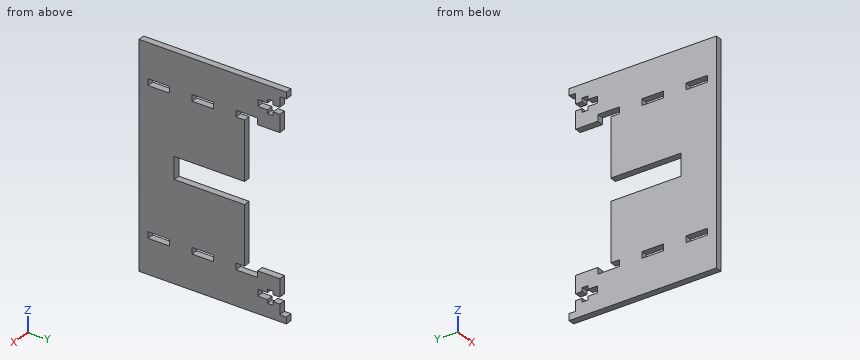
```python
from build123d import *

# Parameters (mm, degrees)
SKETCH1_W           = 100
SKETCH1_H           = 64
BOSS_EXTRUDE1_DEPTH = 3
SKETCH2_W           = 2.9
SKETCH2_H           = 9.8
CUT_EXTRUDE1_DEPTH  = 3
CUT_EXTRUDE2_DEPTH  = 10
SKETCH5_W           = 63
SKETCH5_H           = 16
CUT_EXTRUDE3_DEPTH  = 10
SKETCH6_W           = 10
SKETCH6_H           = 32
CUT_EXTRUDE4_DEPTH  = 10
SKETCH7_W           = 3
SKETCH7_H           = 3
BOSS_EXTRUDE2_DEPTH = 3


with BuildPart() as part:
    # Sketch1 → Boss-Extrude1 (new body)
    with BuildSketch(Plane(origin=(0, 0, 0), x_dir=(0, 0, -1), z_dir=(1, 0, 0))):
        Rectangle(SKETCH1_W, SKETCH1_H)
    extrude(amount=BOSS_EXTRUDE1_DEPTH)

    # Sketch2 → Cut-Extrude1 (cut)
    with BuildSketch(Plane(origin=(3, 0, 0), x_dir=(0, 0, -1), z_dir=(1, 0, 0))):
        with Locations((-32.95, 17)):
            Rectangle(SKETCH2_W, SKETCH2_H)
        with Locations((-32.95, -3)):
            Rectangle(SKETCH2_W, SKETCH2_H)
        with Locations((-32.95, -23)):
            Rectangle(SKETCH2_W, SKETCH2_H)
        with Locations((32.95, -23)):
            Rectangle(SKETCH2_W, SKETCH2_H)
        with Locations((32.95, -3)):
            Rectangle(SKETCH2_W, SKETCH2_H)
        with Locations((32.95, 17)):
            Rectangle(SKETCH2_W, SKETCH2_H)
    extrude(amount=-CUT_EXTRUDE1_DEPTH, mode=Mode.SUBTRACT)

    # Sketch3 → Cut-Extrude2 (cut)
    with BuildSketch(Plane(origin=(3, 0, 0), x_dir=(0, 0, -1), z_dir=(1, 0, 0))):
        Polygon((-42.4, 32), (-42.4, 29), (-44, 29), (-44, 26.4), (-42.4, 26.4), (-42.4, 22), (-39.4, 22), (-39.4, 26.4), (-37.8, 26.4), (-37.8, 29), (-39.4, 29), (-39.4, 32), align=None)
    cut_extrude2 = extrude(amount=-CUT_EXTRUDE2_DEPTH, mode=Mode.SUBTRACT)

    # Mirror1: Cut-Extrude2 across plane
    add(cut_extrude2.mirror(Plane.XY), mode=Mode.SUBTRACT)

    # Sketch5 → Cut-Extrude3 (cut)
    with BuildSketch(Plane(origin=(3, 0, 0), x_dir=(0, 0, -1), z_dir=(1, 0, 0))):
        with Locations((0, 24)):
            Rectangle(SKETCH5_W, SKETCH5_H)
    extrude(amount=-CUT_EXTRUDE3_DEPTH, mode=Mode.SUBTRACT)

    # Sketch6 → Cut-Extrude4 (cut)
    with BuildSketch(Plane(origin=(3, 0, 0), x_dir=(0, 0, -1), z_dir=(1, 0, 0))):
        Rectangle(SKETCH6_W, SKETCH6_H)
    extrude(amount=-CUT_EXTRUDE4_DEPTH, mode=Mode.SUBTRACT)

    # Sketch7 → Boss-Extrude2 (add)
    with BuildSketch(Plane(origin=(3, 0, 0), x_dir=(0, 0, -1), z_dir=(1, 0, 0))):
        with Locations((-48.5, 33.5)):
            Rectangle(SKETCH7_W, SKETCH7_H)
        with Locations((48.5, 33.5)):
            Rectangle(SKETCH7_W, SKETCH7_H)
    extrude(amount=-BOSS_EXTRUDE2_DEPTH)


solid = part.part
```
Design review of the part built by this model. Coordinates are the model's own, in mm. Coordinates: 2 decimals unless noted, no trailing zeros. Order: outer loops, then holes, each group sorted by start corner. A loop starts at its lowest first (then second) coordinate and runs counter-clockwise, first axis right, second up. Notation, with made-up numbers: (50, 11.25) -> (68, 11.25) arc R24 cw to (68, 28.25) -> close; hole circle Ø5 at (0, 34). An arc over 180 degrees is marked (long way). One line per item, written item: value. Start each with the question number.
Q1. Take a section at D-D, the plane z = 13. State the section outline as (x, y) points, then the cut area to 3 significant figures.
Q2. Insertion check: pin 1 Ø1.5 at (x, z) = (1.5, -24.5) entering from +Y. The pin has a flat end and moves straight along its axis. Give the tip position at first contact, or say it passes through.
Q3. Take a section at C-C, the plane x = 1.45. Give the number of separate pieces and of enclosed holes in the cut face, then the cut area to 3 significant figures.
Q4. Take a section at B-B, the plane y = -3. State the section outline as (x, z) points.
Q5. For probe 1 along Z at (x, y) = (2.25, -5); probe 2 along Z at (x, y) = (2.45, 30); probe 3 along Z at (x, y) = (2.55, -27), list the stretches that pass through material, from the lowest coordinate up.
Q6. Take a section at A-A, the plane y = 4.5. State the section outline as (x, z) points, then the cut area to 3 significant figures.
Values follow:
1. outline: (0, -32) -> (3, -32) -> (3, 16) -> (0, 16) -> close
1. area: 144 mm2
2. pin 1: stops at y = 16
3. separate pieces: 1
3. enclosed holes: 4
3. area: 4,840 mm2
4. outline: (0, -50) -> (3, -50) -> (3, -34.4) -> (0, -34.4) -> close; (0, -31.5) -> (3, -31.5) -> (3, -5) -> (0, -5) -> close; (0, 5) -> (3, 5) -> (3, 31.5) -> (0, 31.5) -> close; (0, 34.4) -> (3, 34.4) -> (3, 50) -> (0, 50) -> close
5. probe 1: z = -50 to -34.4, -31.5 to -5, 5 to 31.5, 34.4 to 50
5. probe 2: z = -50 to -42.4, -39.4 to -31.5, 31.5 to 39.4, 42.4 to 50
5. probe 3: z = -50 to -34.4, -31.5 to 31.5, 34.4 to 50
6. outline: (0, -50) -> (3, -50) -> (3, -5) -> (0, -5) -> close; (0, 5) -> (3, 5) -> (3, 50) -> (0, 50) -> close
6. area: 270 mm2
